```python
from build123d import *

# Parameters (mm, degrees)
SKETCH2_W           = 38
SKETCH2_H           = 38
BOSS_EXTRUDE1_DEPTH = 63
SKETCH3_W           = 51
SKETCH3_H           = 10
CUT_EXTRUDE1_DEPTH  = 83.807004535
SKETCH4_W           = 20
SKETCH4_H           = 8
CUT_EXTRUDE2_DEPTH  = 83.807004535
SKETCH5_R           = 16
SKETCH5_R_2         = 14
CUT_EXTRUDE3_DEPTH  = 5
SKETCH6_R           = 3
BOSS_EXTRUDE2_DEPTH = 3
BOSS_EXTRUDE3_START = -21
SKETCH6_2_R         = 3
BOSS_EXTRUDE3_DEPTH = 3
CHAMFER1_SIZE       = 3


with BuildPart() as part:
    # Sketch2 → Boss-Extrude1 (new body)
    with BuildSketch(Plane.XY):
        with Locations((19, 19)):
            Rectangle(SKETCH2_W, SKETCH2_H)
    extrude(amount=-BOSS_EXTRUDE1_DEPTH)

    # Sketch3 → Cut-Extrude1 (cut, through all)
    with BuildSketch(Plane(origin=(38, 0, 0), x_dir=(0, 0, -1), z_dir=(1, 0, 0))):
        with Locations((31.5, 33)):
            Rectangle(SKETCH3_W, SKETCH3_H)
        with Locations((31.5, 5)):
            Rectangle(SKETCH3_W, SKETCH3_H)
    extrude(amount=-CUT_EXTRUDE1_DEPTH, mode=Mode.SUBTRACT)

    # Sketch4 → Cut-Extrude2 (cut, through all)
    with BuildSketch(Plane.XY):
        with Locations((19, 19)):
            Rectangle(SKETCH4_W, SKETCH4_H)
    extrude(amount=-CUT_EXTRUDE2_DEPTH, mode=Mode.SUBTRACT)

    # Sketch5 → Cut-Extrude3 (cut)
    with BuildSketch(Plane.XY):
        with Locations((19, 19)):
            Circle(SKETCH5_R)
        with Locations((19, 19)):
            Circle(SKETCH5_R_2, mode=Mode.SUBTRACT)
    extrude(amount=-CUT_EXTRUDE3_DEPTH, mode=Mode.SUBTRACT)

    # Sketch6 → Boss-Extrude2 (add)
    with BuildSketch(Plane(origin=(0, 28, 0), x_dir=(1, 0, 0), z_dir=(0, 1, 0))):
        with Locations(Location((32, 12, 0), (0, 0, 90))):
            Circle(SKETCH6_R)
        with Locations(Location((32, 22, 0), (0, 0, 90))):
            Circle(SKETCH6_R)
        with Locations(Location((32, 32, 0), (0, 0, 90))):
            Circle(SKETCH6_R)
        with Locations(Location((32, 42, 0), (0, 0, 90))):
            Circle(SKETCH6_R)
        with Locations(Location((32, 52, 0), (0, 0, 90))):
            Circle(SKETCH6_R)
        with Locations(Location((6, 12, 0), (0, 0, 90))):
            Circle(SKETCH6_R)
        with Locations(Location((6, 22, 0), (0, 0, 90))):
            Circle(SKETCH6_R)
        with Locations(Location((6, 32, 0), (0, 0, 90))):
            Circle(SKETCH6_R)
        with Locations(Location((6, 42, 0), (0, 0, 90))):
            Circle(SKETCH6_R)
        with Locations(Location((6, 52, 0), (0, 0, 90))):
            Circle(SKETCH6_R)
    extrude(amount=BOSS_EXTRUDE2_DEPTH)

    # Sketch6<2> → Boss-Extrude3 (add)
    with BuildSketch(Plane(origin=(0, 28, 0), x_dir=(1, 0, 0), z_dir=(0, 1, 0)).offset(BOSS_EXTRUDE3_START)):
        with Locations(Location((32, 12, 0), (0, 0, 90))):
            Circle(SKETCH6_2_R)
        with Locations(Location((32, 22, 0), (0, 0, 90))):
            Circle(SKETCH6_2_R)
        with Locations(Location((32, 32, 0), (0, 0, 90))):
            Circle(SKETCH6_2_R)
        with Locations(Location((32, 42, 0), (0, 0, 90))):
            Circle(SKETCH6_2_R)
        with Locations(Location((32, 52, 0), (0, 0, 90))):
            Circle(SKETCH6_2_R)
        with Locations(Location((6, 12, 0), (0, 0, 90))):
            Circle(SKETCH6_2_R)
        with Locations(Location((6, 22, 0), (0, 0, 90))):
            Circle(SKETCH6_2_R)
        with Locations(Location((6, 32, 0), (0, 0, 90))):
            Circle(SKETCH6_2_R)
        with Locations(Location((6, 42, 0), (0, 0, 90))):
            Circle(SKETCH6_2_R)
        with Locations(Location((6, 52, 0), (0, 0, 90))):
            Circle(SKETCH6_2_R)
    extrude(amount=BOSS_EXTRUDE3_DEPTH)

    # Chamfer1
    chamfer1_edges = [part.edges().sort_by_distance(p)[0] for p in [
        (0, 0, -3),
        (38, 0, -3),
        (38, 38, -3),
        (0, 38, -3),
        (0, 38, -60),
        (38, 38, -60),
        (38, 0, -60),
        (0, 0, -60),
    ]]
    chamfer(chamfer1_edges, length=CHAMFER1_SIZE)


solid = part.part
```
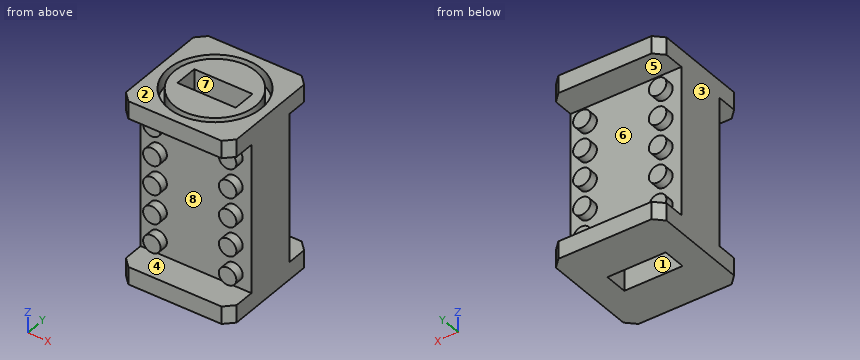
Model file for the job. Use its own axes, mm. Face numbers are marked on the shaded views. A direction names the side the tool comes from. Give positions to 0.01 mm unless a question says otherwise; leave off trailing zeros. Loops run counter-clockwise (first coordinate to the right, second up) from the corner with the lowest first, then second, coordinate; pieces in that order, holes last. Notation, with made-up numbers: (6.5, 2.5) -> (37.5, 2.5) arc R26 cw to (37.5, 37.5) -> close; hole circle Ø11 at (62, 13.5). An arc over 180 degrees is marked (long way). Use CSV: the item, a comma, the result in double quotes. Start each with the question number.
1) Slice it at D-D on y = 8. Give the number of separate pieces and of enclosed holes in the cut face, plus the area to 3 significant figures.
2) Mould opens along X. For the marked faces 1, 2 and 3 say: released by +X, released by -X, zero draft, split by the parting line, or undercut.
3) Flat gauge pins, fed straight in: pin 1 Ø6.5 at (x, z) = (7.5, -42) entering from -Y; pin 2 Ø4 at (x, z) = (18, -20) entering from +Y; pin 3 Ø6.5 at (x, z) = (32.5, -50.5) entering from +Y. Where does each tip first touch, or does it go through?
4) Tool access for the marked faces 4, 5, 6, 7 and 8: list every direction of +Z, -Z, +X, -X, +Y, -Y with a clear straight run to the whole face (end or side of a thin tool).
5) Slice it at B-B on z = -52. Give the cut face in (x, y).
6) Wall check: line 1 (Y direction, x = 19, z = -3); line 2 (X direction, y = 22.5, z = -44); line 3 (Z direction, x = 8, y = 5). Give the ranges that are in metal, low to high.
7) Slice it at C-C on y = 19. Give the cut face in (x, z), plus the area to 3 significant figures.
8) Slice it at A-A on x = 19. Give the cut face in (y, z).
Computed values:
1,separate pieces,"12"
1,enclosed holes,"0"
1,area,"709 mm^2"
2,face 1,"undercut"
2,face 2,"zero draft"
2,face 3,"released by -X"
3,pin 1,"stops at y = 7"
3,pin 2,"stops at y = 28"
3,pin 3,"stops at y = 31"
4,face 4,"+X, -X, -Y"
4,face 5,"+X, -X, +Y"
4,face 6,"+Y"
4,face 7,"+Z, -Z"
4,face 8,"-Y"
5,outline,"(0, 10) -> (3, 10) -> (3, 7) -> (9, 7) -> (9, 10) -> (29, 10) -> (29, 7) -> (35, 7) -> (35, 10) -> (38, 10) -> (38, 28) -> (35, 28) -> (35, 31) -> (29, 31) -> (29, 28) -> (9, 28) -> (9, 31) -> (3, 31) -> (3, 28) -> (0, 28) -> close; hole (9, 15) -> (29, 15) -> (29, 23) -> (9, 23) -> close"
6,line 1,"y = 0 to 3, 5 to 15, 23 to 33, 35 to 38"
6,line 2,"x = 0 to 9, 29 to 38"
6,line 3,"z = -63 to -57, -6 to 0"
7,outline,"(0, -63) -> (9, -63) -> (9, 0) -> (5, 0) -> (5, -5) -> (3, -5) -> (3, 0) -> (0, 0) -> close; (29, -63) -> (38, -63) -> (38, 0) -> (35, 0) -> (35, -5) -> (33, -5) -> (33, 0) -> (29, 0) -> close"
7,area,"1,110 mm^2"
8,outline,"(0, -63) -> (15, -63) -> (15, 0) -> (5, 0) -> (5, -5) -> (3, -5) -> (3, 0) -> (0, 0) -> (0, -6) -> (10, -6) -> (10, -57) -> (0, -57) -> close; (23, -63) -> (38, -63) -> (38, -57) -> (28, -57) -> (28, -6) -> (38, -6) -> (38, 0) -> (35, 0) -> (35, -5) -> (33, -5) -> (33, 0) -> (23, 0) -> close"
